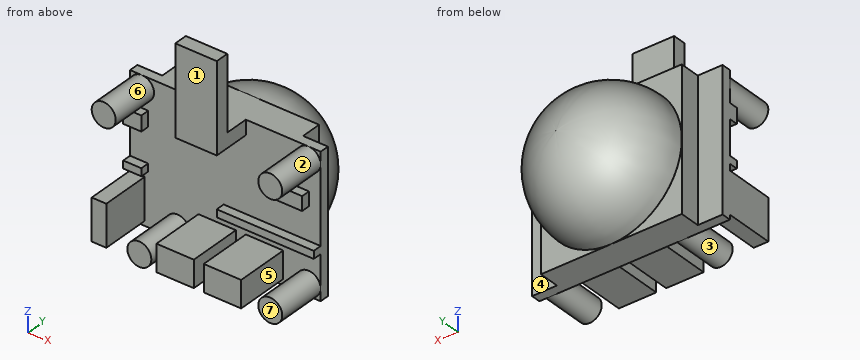
from build123d import *

# Parameters (mm, degrees)
F2_DEPTH  = 1.6
F3_DEPTH  = 5.1
F4_DEPTH  = 17.2
F1_R      = 2.05
F1_W      = 2.5
F1_H      = 7.1
F6_DEPTH  = 8.4
F1_W_2    = 6.4
F1_H_2    = 4.6
F7_DEPTH  = 9.2
F1_W_3    = 3.1
F1_H_3    = 1.3
F1_W_4    = 4.6
F1_H_4    = 2.4
F1_W_5    = 16.6
F1_H_5    = 2.6
F8_DEPTH  = 1.5
F1_W_6    = 7.1
F1_H_6    = 2.5
F9_DEPTH  = 6.35
F10_W     = 7.1
F10_H     = 2.3
F11_DEPTH = 12.7


# Not quite as in the source:
# - a fillet or chamfer that OpenCascade refuses, or shapes differently, is made with other operations: its cross-section is extruded or revolved along the edge and cut away or added


with BuildPart() as f2:
    # F0 (on Front) → F2 (new body)
    with BuildSketch(Plane.XZ):
        Polygon((16.3, -12.05), (16.3, 12.05), (12.05, 12.05), (12.05, 0), (12.05, -12.05), align=None)
        with BuildLine():
            Line((12.05, 0), (12.05, 12.05))
            Line((12.05, 12.05), (0, 12.05))
            ThreePointArc((0, 12.05), (8.5206367133, 8.5206367133), (12.05, 0))
        make_face()
        with BuildLine():
            ThreePointArc((-12.05, 0), (-8.5206367133, 8.5206367133), (0, 12.05))
            Line((0, 12.05), (-12.05, 12.05))
            Line((-12.05, 12.05), (-12.05, 0))
        make_face()
        with BuildLine():
            ThreePointArc((12.05, 0), (8.5206367133, 8.5206367133), (0, 12.05))
            ThreePointArc((0, 12.05), (-8.5206367133, 8.5206367133), (-12.05, 0))
            ThreePointArc((-12.05, 0), (-8.5206367125, -8.5206367141), (2.1e-09, -12.05))
            ThreePointArc((2.1e-09, -12.05), (8.5206367141, -8.5206367125), (12.05, 0))
        make_face()
        with BuildLine():
            Line((12.05, -12.05), (12.05, 0))
            ThreePointArc((12.05, 0), (8.5206367141, -8.5206367125), (2.1e-09, -12.05))
            Line((2.1e-09, -12.05), (12.05, -12.05))
        make_face()
        Polygon((-12.05, 0), (-12.05, 12.05), (-16.3, 12.05), (-16.3, -12.05), (-12.05, -12.05), align=None)
        with BuildLine():
            ThreePointArc((2.1e-09, -12.05), (-8.5206367125, -8.5206367141), (-12.05, 0))
            Line((-12.05, 0), (-12.05, -12.05))
            Line((-12.05, -12.05), (2.1e-09, -12.05))
        make_face()
    extrude(amount=-F2_DEPTH)

    # F0 (on Front) → F3 (join)
    with BuildSketch(Plane.XZ):
        with BuildLine():
            ThreePointArc((2.1e-09, -12.05), (-8.5206367125, -8.5206367141), (-12.05, 0))
            Line((-12.05, 0), (-12.05, -12.05))
            Line((-12.05, -12.05), (2.1e-09, -12.05))
        make_face()
        with BuildLine():
            ThreePointArc((-12.05, 0), (-8.5206367133, 8.5206367133), (0, 12.05))
            Line((0, 12.05), (-12.05, 12.05))
            Line((-12.05, 12.05), (-12.05, 0))
        make_face()
        with BuildLine():
            ThreePointArc((12.05, 0), (8.5206367133, 8.5206367133), (0, 12.05))
            ThreePointArc((0, 12.05), (-8.5206367133, 8.5206367133), (-12.05, 0))
            ThreePointArc((-12.05, 0), (-8.5206367125, -8.5206367141), (2.1e-09, -12.05))
            ThreePointArc((2.1e-09, -12.05), (8.5206367141, -8.5206367125), (12.05, 0))
        make_face()
        with BuildLine():
            Line((12.05, 0), (12.05, 12.05))
            Line((12.05, 12.05), (0, 12.05))
            ThreePointArc((0, 12.05), (8.5206367133, 8.5206367133), (12.05, 0))
        make_face()
        with BuildLine():
            Line((12.05, -12.05), (12.05, 0))
            ThreePointArc((12.05, 0), (8.5206367141, -8.5206367125), (2.1e-09, -12.05))
            Line((2.1e-09, -12.05), (12.05, -12.05))
        make_face()
    extrude(amount=-F3_DEPTH)

    # F0 (on Front) → F4 (join)
    with BuildSketch(Plane.XZ):
        with BuildLine():
            ThreePointArc((12.05, 0), (8.5206367133, 8.5206367133), (0, 12.05))
            ThreePointArc((0, 12.05), (-8.5206367133, 8.5206367133), (-12.05, 0))
            ThreePointArc((-12.05, 0), (-8.5206367125, -8.5206367141), (2.1e-09, -12.05))
            ThreePointArc((2.1e-09, -12.05), (8.5206367141, -8.5206367125), (12.05, 0))
        make_face()
    extrude(amount=-F4_DEPTH)

    # F5: fillet of radius 12 on 1 edges, made by hand

    # F5_s1 → F5_t2 (revolve, cut)
    with BuildSketch(Plane.YZ):
        with BuildLine():
            ThreePointArc((5.2, -12.05), (13.6852813742, -8.5352813742), (17.2, -0.05))
            Line((17.2, -0.05), (17.2, -12.05))
            Line((17.2, -12.05), (5.2, -12.05))
        make_face()
    revolve(axis=Axis((0, 17.2, 0), (0, -1, 0)), mode=Mode.SUBTRACT)

    # F1 (on Front) → F6 (join)
    with BuildSketch(Plane.XZ):
        with Locations((-14.25, 10)):
            Circle(F1_R)
        with Locations((14.25, 10)):
            Circle(F1_R)
        with Locations((14.25, -10)):
            Circle(F1_R)
        with Locations((-8.15, -10)):
            Circle(F1_R)
        with Locations((-15.05, -7.7)):
            Rectangle(F1_W, F1_H)
    extrude(amount=F6_DEPTH)

    # F1 (on Front) → F7 (join)
    with BuildSketch(Plane.XZ):
        with Locations((-1.4, -8.75)):
            Rectangle(F1_W_2, F1_H_2)
        with Locations((6.7, -8.75)):
            Rectangle(F1_W_2, F1_H_2)
    extrude(amount=F7_DEPTH)

    # F1 (on Front) → F8 (join)
    with BuildSketch(Plane.XZ):
        with Locations((-14.75, -2.4)):
            Rectangle(F1_W_3, F1_H_3)
        with Locations((12, 3.65)):
            Rectangle(F1_W_4, F1_H_4)
        with Locations((8, -3.8)):
            Rectangle(F1_W_5, F1_H_3)
        with Locations((-14.75, 5.45)):
            Rectangle(F1_W_3, F1_H_5)
    extrude(amount=F8_DEPTH)

    # F1 (on Front) → F9 (join)
    with BuildSketch(Plane.XZ):
        with Locations((-0.05, 10.8)):
            Rectangle(F1_W_6, F1_H_6)
    extrude(amount=F9_DEPTH)

    # F10 (on face) → F11 (join)
    with BuildSketch(Plane.XY.offset(12.05)):
        with Locations((-0.05, -5.2)):
            Rectangle(F10_W, F10_H)
    extrude(amount=F11_DEPTH)


solid = f2.part
Source: CAD feature listing. Evaluate the final solid. Frame: model axes, mm. Face numbers are marked on the shaded views. A direction names the side the tool comes from. Give positions to 0.01 mm unless a question says otherwise; leave off trailing zeros. Write each loop counter-clockwise with the first axis right and the second up, starting at its lowest first coordinate (ties: lowest second). Pieces come first, ordered by that corner, then holes. Notation, with made-up numbers: M 48,-3.75 L 71,-3.75 A21 ccw 71,8.25 Z; hole C 63,83 d8. An arc over 180 degrees is marked long. Answer as a JSON object with one key per item and string values.
Q1. Access query for the marked faces 4, 5, 6 and 7. Directions: +Z, -Z, +X, -X, +Y, -Y. A direction counts if a zero-diameter tool reaches every point of the face in a straight line with its end or side. Return the directions, or none.
Geometry check:
{"face 4": "+Z, -Z, +X, +Y", "face 5": "-Z, -Y", "face 6": "-Y", "face 7": "+Z, -Z, +X, -Y"}
Q2. Cut plane C-C, the plane y = 2.5. Return the cut outline in (x, z), then the cut area to 3 significant figures.
Geometry check:
{"outline": "M -12.05,-12.05 L 12.05,-12.05 L 12.05,12.05 L -12.05,12.05 Z", "area": "581 mm^2"}
Q3. Mould query, pull axis Z, two halves, no side actions, for the marked faces 1, 2 and 3. Classes: +Z half, -Z half, draft (parallel to the pull), parting line (faces both ways), or undercut.
Geometry check:
{"face 1": "draft", "face 2": "undercut", "face 3": "parting line"}
Q4. Contact query for flat-ended pins moving along their axis: P1, Ø7, axis at y = -4, z = 20.5, coming from the -X side; P2, Ø1, axis at x = 0, y = -0.5, coming from the +Z side; P3, Ø2, axis at x = -7.5, y = 7.5, coming from the -Z side. Output: stop coordinate, or through.
Geometry check:
{"P1": "stops at x = -3.6", "P2": "stops at z = 12.05", "P3": "stops at z = -9.92"}
Q5. Cut plane A-A, the plane y = -5.75. Return the cut outline in (x, z), then the cut area to 3 significant figures.
Geometry check:
{"outline": "M -16.3,-11.25 L -13.8,-11.25 L -13.8,-4.15 L -16.3,-4.15 Z; C -14.25,10 d4.1; C -8.15,-10 d4.1; M -4.6,-11.05 L 1.8,-11.05 L 1.8,-6.45 L -4.6,-6.45 Z; M -3.6,9.55 L 3.5,9.55 L 3.5,24.75 L -3.6,24.75 Z; M 3.5,-11.05 L 9.9,-11.05 L 9.9,-6.45 L 3.5,-6.45 Z; C 14.25,-10 d4.1; C 14.25,10 d4.1", "area": "237 mm^2"}
Q6. Cut plane B-B, the plane z = 19. Return the cut outline in (x, y).
Geometry check:
{"outline": "M -3.6,-6.35 L 3.5,-6.35 L 3.5,-4.05 L -3.6,-4.05 Z"}
Q7. Ray query, line 1 along Y through (x, z) = (-13, -8); line 2 along Y through (x, z) = (-11.5, 9.5); line 3 along Z through (x, y) = (-8, -7). Return the intervals inside material, ascending.
Geometry check:
{"line 1": "y = 0 to 1.6", "line 2": "y = 0 to 5.1", "line 3": "z = -12.04 to -7.96"}
